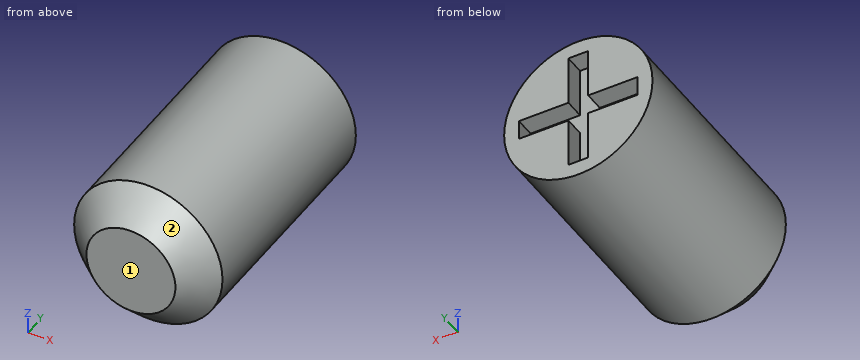
Autodesk Inventor part; units mm, degrees
ref_plane "YZ Plane" through (0, 0, 0) normal (1, 0, 0) x (0, 1, 0)
ref_plane "XZ Plane" through (0, 0, 0) normal (0, 1, 0) x (-1, 0, 0)
ref_plane "XY Plane" through (0, 0, 0) normal (0, 0, 1) x (1, 0, 0)
sketch "Esquisse1" plane through (0, 0, 0) normal (0, 1, 0) x (-1, 0, 0)
  circle A0 centre (0, 0) radius 7.5
  dimension "d0" = 15
extrude "Extrusion1" add sketch "Esquisse1" along normal blind 26
chamfer "Chanfrein1" distance 3 angle 45 1 edges at (7.5, 0, 0)
sketch "Esquisse2" plane through (0, 26, 0) normal (0, 1, 0) x (1, 0, 0)
  line L0 (6, -1) -> (6, 1)
  line L1 (-6, 1) -> (-6, -1)
  line L2 (-1, -6) -> (1, -6)
  line L3 (1, 6) -> (-1, 6)
  circle A0 centre (0, 0) radius 7.5
  line L4 (-1, 6) -> (-1, 1)
  line L5 (-1, -1) -> (-1, -6)
  line L6 (1, -6) -> (1, -1)
  line L7 (1, 1) -> (1, 6)
  line L8 (6, 1) -> (1, 1)
  line L9 (-1, 1) -> (-6, 1)
  line L10 (-6, -1) -> (-1, -1)
  line L11 (1, -1) -> (6, -1)
  circle A1 centre (0, 0) radius 4.5
  dimension "d6" = 6
  dimension "d7" = 6
  dimension "d8" = 6
  dimension "d9" = 6
  dimension "d16" = 1
  dimension "d17" = 1
  dimension "d18" = 1
  dimension "d19" = 1
  dimension "d20" = 1
  dimension "d21" = 1
  dimension "d22" = 1
  dimension "d23" = 1
extrude "Extrusion2" cut sketch "Esquisse2" against normal blind 2 contours L11 A1 L8 L0 | L11 L6 A1 L5 L10 L9 L4 L7 L8 | L6 L2 L5 A1 | A1 L4 L3 L7 | L10 L1 L9 A1
sketch "Esquisse3" plane through (0, 24, 0) normal (0, 1, 0) x (1, 0, 0)
  point P0 (0, 0)
properties part number "Pion croix"
Design review of the part built by this model. Coordinates are the model's own, in mm. Face numbers are marked on the shaded views. Coordinates: 2 decimals unless noted, no trailing zeros. Order: outer loops, then holes, each group sorted by start corner. A loop starts at its lowest first (then second) coordinate and runs counter-clockwise, first axis right, second up.
Item 1: Take a section at D-D, the plane y = 18. Write out the cut boundary in (x, z).
Item 2: Take a section at B-B, the plane z = 0. Write out the cut boundary in (x, y), then the cut area to 3 significant figures.
Item 3: For line 1 (Z direction, x = 6, y = 7); line 2 (X direction, y = 10.5, z = -4.5), list the stretches that pass through material, from the lowest coordinate up.
Item 4: The part is to be moulded in two halves that separate along X. For the marked faces 1 and 2, say which applies: pulls with the +X half, pulls with the -X half, needs draft (parallel to the pull), parting line crosses it, or undercut.
Item 5: Take a section at A-A, the plane x = 0. Write out the cut boundary in (y, z), then the cut area to 3 significant figures.
Item 6: Take a section at C-C, the plane y = 2.25. Write out the cut boundary in (x, z), then the cut area to 3 significant figures.
Item 7: For pin 1 Ø1.6 at (x, y) = (3, 25) entering from -Z; pin 2 Ø1.5 at (x, z) = (-2.5, -5.5) entering from -Y; pin 3 Ø1.6 at (y, z) = (25.5, 3) entering from -X; pin 4 Ø1.6 at (y, z) = (25, -0.5) entering from +X, all flat-tipped, find the tip position at first contact; note any pin that passes through.
The answers:
1. outline: circle Ø15 at (0, 0)
2. outline: (-7.5, 3) - (-4.5, 0) - (4.5, 0) - (7.5, 3) - (7.5, 26) - (6, 26) - (6, 24) - (-6, 24) - (-6, 26) - (-7.5, 26) - close
2. area: 357 mm2
3. line 1: z = -4.5 to 4.5
3. line 2: x = -6 to 6
4. face 1: needs draft
4. face 2: parting line crosses it
5. outline: (0, -4.5) - (3, -7.5) - (26, -7.5) - (26, -6) - (24, -6) - (24, 6) - (26, 6) - (26, 7.5) - (3, 7.5) - (0, 4.5) - close
5. area: 357 mm2
6. outline: circle Ø13.5 at (0, 0)
6. area: 143 mm2
7. pin 1: stops at z = -7.17
7. pin 2: stops at y = 0.79
7. pin 3: stops at x = -7.17
7. pin 4: stops at x = 7.5
